```python
from build123d import *

# Parameters (mm, degrees)
SKETCH1_W                          = 660.4
SKETCH1_H                          = 179.07
BASE_FLANGE1_DEPTH                 = 1.5875
MITER_START                        = -330.2
MITER_FLANGE1_DEPTH                = 660.4
MITER_FLANGE1_2_DEPTH              = 660.4
F_3_16_0_1875_DIAMETER_HOLE1_D     = 4.7625
F_3_16_0_1875_DIAMETER_HOLE1_DEPTH = 5.1054
F_3_16_0_1875_DIAMETER_HOLE1_TIP   = 1.430799349
SKETCH25_R                         = 3.2639
CUT_EXTRUDE1_DEPTH                 = 346.837375989
FILLET1_R                          = 3.175


# Read off the part's stored shape, not the designer's step: Miter Flange1
# Sheet-metal steps are written as plain solids
with BuildPart() as part:
    # Sketch1 → Base-Flange1 (new body)
    with BuildSketch(Plane.XY):
        Rectangle(SKETCH1_W, SKETCH1_H)
    extrude(amount=-BASE_FLANGE1_DEPTH)

    # Miter Flange1 outline → Miter Flange1 (cut)
    with BuildSketch(Plane.YZ.offset(MITER_START)):
        with BuildLine():
            ThreePointArc((87.9475, 0), (88.769250468, -0.108185502), (89.535, -0.425369343))
            Line((89.535, -0.425369343), (89.535, 0))
            Line((89.535, 0), (87.9475, 0))
        make_face()
    miter_flange1 = extrude(amount=MITER_FLANGE1_DEPTH, mode=Mode.SUBTRACT)

    # Miter Flange1 2 outline → Miter Flange1 2 (add)
    with BuildSketch(Plane.YZ.offset(MITER_START)):
        with BuildLine():
            Line((87.9475, -46.0375), (64.135, -46.0375))
            Line((64.135, -46.0375), (64.135, -47.625))
            Line((64.135, -47.625), (87.9475, -47.625))
            ThreePointArc((87.9475, -47.625), (90.19256403, -46.69506403), (91.1225, -44.45))
            Line((91.1225, -44.45), (91.1225, -3.175))
            ThreePointArc((91.1225, -3.175), (90.697130657, -1.5875), (89.535, -0.425369343))
            Line((89.535, -0.425369343), (89.535, -1.5875))
            Line((89.535, -1.5875), (87.9475, -1.5875))
            ThreePointArc((87.9475, -1.5875), (89.070032015, -2.052467985), (89.535, -3.175))
            Line((89.535, -3.175), (89.535, -44.45))
            ThreePointArc((89.535, -44.45), (89.070032015, -45.572532015), (87.9475, -46.0375))
        make_face()
    miter_flange1_2 = extrude(amount=MITER_FLANGE1_2_DEPTH)

    # Mirror1: Miter Flange1, Miter Flange1 2 across plane
    add(miter_flange1.mirror(Plane.ZX), mode=Mode.SUBTRACT)
    add(miter_flange1_2.mirror(Plane.ZX))

    # 3/16 (0.1875) Diameter Hole1
    with Locations(Plane(origin=(0, 0, -47.625), x_dir=(-1, 0, 0), z_dir=(0, 0, -1))):
        with Locations((-292.1, 82.55), (-292.1, -82.55), (-97.366666667, 82.55), (-97.366666667, -82.55), (97.366666667, 82.55), (97.366666667, -82.55), (292.1, -82.55), (292.1, 82.55)):
            Hole(F_3_16_0_1875_DIAMETER_HOLE1_D / 2, depth=F_3_16_0_1875_DIAMETER_HOLE1_DEPTH)
            with Locations((0, 0, -(F_3_16_0_1875_DIAMETER_HOLE1_DEPTH + F_3_16_0_1875_DIAMETER_HOLE1_TIP / 2))):  # 118° drill point
                Cone(0, F_3_16_0_1875_DIAMETER_HOLE1_D / 2, F_3_16_0_1875_DIAMETER_HOLE1_TIP, mode=Mode.SUBTRACT)

    # Sketch25 → Cut-Extrude1 (cut, through all)
    with BuildSketch(Plane.XY):
        with Locations((47.625, 47.625)):
            Circle(SKETCH25_R)
        with Locations((47.625, -47.625)):
            Circle(SKETCH25_R)
        with Locations((-47.625, -47.625)):
            Circle(SKETCH25_R)
        with Locations((-47.625, 47.625)):
            Circle(SKETCH25_R)
    extrude(amount=-CUT_EXTRUDE1_DEPTH, mode=Mode.SUBTRACT)

    # Fillet1
    fillet1_edges = [part.edges().sort_by_distance(p)[0] for p in [
        (330.2, 64.135, -46.83125),
        (-330.2, 64.135, -46.83125),
        (330.2, -64.135, -46.83125),
        (-330.2, -64.135, -46.83125),
    ]]
    fillet(fillet1_edges, radius=FILLET1_R)


solid = part.part
```
Geometry check sheet. Reference: the model listing, model coordinates, mm. A direction names the side the tool comes from. Coordinates: 2 decimals unless noted, no trailing zeros. Order: outer loops, then holes, each group sorted by start corner. A loop starts at its lowest first (then second) coordinate and runs counter-clockwise, first axis right, second up.
Item 1: Tool access check on faces 1 (the flat face through (-5, 91.122, -24)), 2 (the flat face through (-5, -89.535, -24)). Record the directions out of +Z, -Z, +X, -X, +Y, -Y that give a thin tool (end or side, any length) a straight path to the whole face; none if there is none.
Item 2: Section check C-C (y = 24). Enter the section's corners in (x, z).
Item 3: Scan lines: line 1 along Y through (x, z) = (46, -44.5); line 2 along Y through (x, z) = (292.1, -47.2) (3 decimals); line 3 along Z through (x, y) = (-178, -80.5) (1 decimal). Record each from-to range of solid material in increasing order.
Item 4: Mould release check, pull along Z, two halves, no side actions. Record for faces 3 (the flat face through (-5, 1, -1.588)), 4 (the flat face through (-5, 76, -47.625)), 5 (the flat face through (-330.2, 0, -1)): released by +Z, released by -Z, zero draft, split by the parting line, or undercut.
Item 5: Section check A-A (z = -19). Enter the section's corners in (x, y) (1 decimal), plus the area to 3 significant figures.
Item 6: Depth check by flat-ended pin: pin 1 (6 mm diameter, centred on x = -47.625, y = -47.625, fed in from -Z); pin 2 (5 mm diameter, centred on x = -193.5, y = -19, fed in from -Z); pin 3 (1.3 mm diameter, centred on x = -34, z = -47, fed in from +Y); pin 4 (0.5 mm diameter, centred on x = -127, z = -46.5, fed in from -Y). Enter the tip coordinate at first touch or a pass-through.
Check sheet entries:
1. face 1: +Z, -Z, +X, -X, +Y
1. face 2: +X, -X
2. outline: (-330.2, -1.59) - (330.2, -1.59) - (330.2, 0) - (-330.2, 0) - close
3. line 1: y = -91.12 to -89.53, 89.53 to 91.12
3. line 2: y = -89.534 to -84.931, -80.169 to -64.135, 64.135 to 80.169, 84.931 to 89.534
3. line 3: z = -47.6 to -46, -1.6 to 0
4. face 3: undercut
4. face 4: released by -Z
4. face 5: zero draft
5. outline: (-330.2, -91.1) - (330.2, -91.1) - (330.2, -89.5) - (-330.2, -89.5) - close; (-330.2, 89.5) - (330.2, 89.5) - (330.2, 91.1) - (-330.2, 91.1) - close
5. area: 2,100 mm2
6. pin 1: passes through
6. pin 2: stops at z = -1.59
6. pin 3: stops at y = 90.49
6. pin 4: stops at y = -90.56
